For this review, take the finished solid that the model builds, in its own axes (mm). A direction names the side the tool comes from. Give positions to 0.01 mm unless a question says otherwise; leave off trailing zeros. Loops run counter-clockwise (first coordinate to the right, second up) from the corner with the lowest first, then second, coordinate; pieces in that order, holes last.
Autodesk Fusion 360 part; units mm, degrees
sketch "Esquisse1" plane through (0, 0, 0) normal (0, 1, 0) x (1, 0, 0)
  line L0 (4.75, 5.5) -> (-4.75, 5.5)
  line L1 (-4.75, 5.5) -> (-4.75, -5.5)
  line L2 (-4.75, -5.5) -> (4.75, -5.5)
  line L3 (4.75, -5.5) -> (4.75, 5.5)
  line L4 (4.75, 5.5) -> (-4.75, -5.5) construction
  line L5 (-4.75, 5.5) -> (4.75, -5.5) construction
  dimension "d1" = 11
  dimension "d2" = 9.5
extrude "Extrusion1" add sketch "Esquisse1" along normal blind 7
sketch "Esquisse2" plane through (0, 7, 0) normal (0, 1, 0) x (-1, 0, 0)
  line L0 (-4.75, 5.5) -> (-4.75, -5.5)
  line L1 (-4.75, -5.5) -> (4.75, -5.5)
  line L2 (4.75, -5.5) -> (4.75, 5.5)
  line L3 (4.75, 5.5) -> (-4.75, 5.5)
  circle A0 centre (0, -0.5) radius 3.5
  dimension "d5" = 7
  dimension "d27" = 5
extrude "Extrusion2" add sketch "Esquisse2" along normal blind 5 contours A0
sketch "Esquisse3" plane through (0, 12, 0) normal (0, 1, 0) x (-1, 0, 0)
  circle A0 centre (0, -0.5) radius 3.5
  circle A1 centre (0, -0.5) radius 3
  dimension "d8" = 6
extrude "Extrusion3" add sketch "Esquisse3" along normal blind 10 contours A1
sketch "Esquisse4" plane through (0, 22, 0) normal (0, 1, 0) x (-1, 0, 0)
  circle A0 centre (0, -0.5) radius 3
  circle A1 centre (0, -0.5) radius 3
  line L0 (0.6, -3.4394) -> (0.6, 2.4394)
  line L1 (-0.6, -3.4394) -> (-0.6, 2.4394)
  dimension "d11" = 0.6
  dimension "d12" = 0.6
extrude "Extrusion4" cut sketch "Esquisse4" against normal blind 8 contours A0 A1 L0 L1
fillet "Congé1" radius 1 2 edges at (-3, 22, -0.5) (3, 22, -0.5)
sketch "Esquisse5" plane through (0, 0, 5.5) normal (0, 0, 1) x (1, 0, 0)
  line L0 (-4.75, 0) -> (4.75, 0)
  line L1 (4.75, 0) -> (4.75, 7)
  line L2 (4.75, 7) -> (-4.75, 7)
  line L3 (-4.75, 7) -> (-4.75, 0)
  line L4 (0.5041, 2.125) -> (-0.4959, 2.125)
  line L5 (-0.4959, 2.125) -> (-0.4959, 1.875)
  line L6 (-0.4959, 1.875) -> (0.5041, 1.875)
  line L7 (0.5041, 1.875) -> (0.5041, 2.125)
  line L8 (0.5041, 2.125) -> (-0.4959, 1.875) construction
  line L9 (-0.4959, 2.125) -> (0.5041, 1.875) construction
  line L10 (0, 0) -> (0, 7) construction
  line L11 (-3.4959, 1.875) -> (-2.4959, 1.875)
  line L12 (-3.4959, 2.125) -> (-3.4959, 1.875)
  line L13 (-2.4959, 2.125) -> (-3.4959, 2.125)
  line L14 (-2.4959, 2.125) -> (-3.4959, 1.875) construction
  line L15 (-2.4959, 1.875) -> (-2.4959, 2.125)
  line L16 (-3.4959, 2.125) -> (-2.4959, 1.875) construction
  line L17 (2.5041, 1.875) -> (3.5041, 1.875)
  line L18 (2.5041, 2.125) -> (2.5041, 1.875)
  line L19 (3.5041, 2.125) -> (2.5041, 2.125)
  line L20 (3.5041, 2.125) -> (2.5041, 1.875) construction
  line L21 (3.5041, 1.875) -> (3.5041, 2.125)
  line L22 (2.5041, 2.125) -> (3.5041, 1.875) construction
  point P0 (0.0041, 2)
  dimension "d18" = 1
  dimension "d19" = 0.25
  dimension "d20" = 2
  dimension "d23" = 3
  dimension "d24" = 0
extrude "Extrusion5" add sketch "Esquisse5" along normal blind 2 contours L4 L5 L6 L7 | L11 L12 L13 L15 | L17 L18 L19 L21
Item 1: Take a section at D-D on y = 1.5. Give the boundary of the cut face in (x, z).
Answer:
outline: (-4.75, -5.5) - (4.75, -5.5) - (4.75, 5.5) - (-4.75, 5.5) - close
Item 2: Tool access review of faces 1 (the flat face through (0, 3, -5.5)), 2 (the flat face through (3, 2.125, 6)), 3 (the cylindrical face through (-1.384, 16.93, 2.162)), 4 (the flat face through (0, 1.875, 6)), 5 (the flat face through (0.6, 18, -1)): name each direction out of +Z, -Z, +X, -X, +Y, -Y from which nothing blocks a thin tool from reaching the whole face with its end or side.
Answer:
face 1: -Z, +X, -X, +Y, -Y
face 2: +Z, +X, -X, +Y
face 3: +Y
face 4: +Z, +X, -X, -Y
face 5: +Z, -Z, +Y
Item 3: Take a section at B-B on x = 0. Give the boundary of the cut face in (y, z) (3 decimals), and give its area (4 significant figures).
Answer:
outline: (0, -5.5) - (7, -5.5) - (7, -4) - (12, -4) - (12, -3.5) - (14, -3.5) - (14, 2.5) - (12, 2.5) - (12, 3) - (7, 3) - (7, 5.5) - (2.125, 5.5) - (2.125, 7.5) - (1.875, 7.5) - (1.875, 5.5) - (0, 5.5) - close
area: 124.5 mm2
Item 4: The part is to be moulded in two halves that separate along X. For faces 6 (the cylindrical face through (-3.34, 9.46, -1.55)), 7 (the flat face through (4.75, 3, 0)), 8 (the flat face through (0, 14, 0)), 9 (the flat face through (3, 1.875, 6)), say which applies: released by +X, released by -X, zero draft, split by the parting line, or undercut.
Answer:
face 6: split by the parting line
face 7: released by +X
face 8: undercut
face 9: zero draft
Item 5: Take a section at A-A on z = 6. Give the boundary of the cut face in (x, y) (3 decimals).
Answer:
outline: (-3.496, 1.875) - (-2.496, 1.875) - (-2.496, 2.125) - (-3.496, 2.125) - close; (-0.496, 1.875) - (0.504, 1.875) - (0.504, 2.125) - (-0.496, 2.125) - close; (2.504, 1.875) - (3.504, 1.875) - (3.504, 2.125) - (2.504, 2.125) - close
Item 6: For L1, parallel to Y at x = -1.5, z = 2.75; L2, parallel to Y at x = -3, z = 6.5 (3 decimals); L3, parallel to Z at x = 0, y = 6, list the stretches that pass through material, from the lowest coordinate up.
Answer:
L1: y = 0 to 7
L2: y = 1.875 to 2.125
L3: z = -5.5 to 5.5
Item 7: Clearance check with flat-ended pins moving along their axes: pin 1 Ø3 at (y, z) = (18.5, -1.5) entering from -X; pin 2 Ø0.6 at (x, z) = (0, 1) entering from +Y; pin 3 Ø3 at (y, z) = (16, -4) entering from +X. State where each tip first meets the part, or that it passes through.
Answer:
pin 1: stops at x = -3
pin 2: stops at y = 14
pin 3: stops at x = 2.24
Item 8: Take a section at C-C on z = -0.5. Give the boundary of the cut face in (x, y), and give its area (3 significant figures).
Answer:
outline: (-4.75, 0) - (4.75, 0) - (4.75, 7) - (3.5, 7) - (3.5, 12) - (3, 12) - (3, 21) arc R1 ccw to (2, 22) - (0.6, 22) - (0.6, 14) - (-0.6, 14) - (-0.6, 22) - (-3, 22) - (-3, 12) - (-3.5, 12) - (-3.5, 7) - (-4.75, 7) - close
area: 152 mm2
